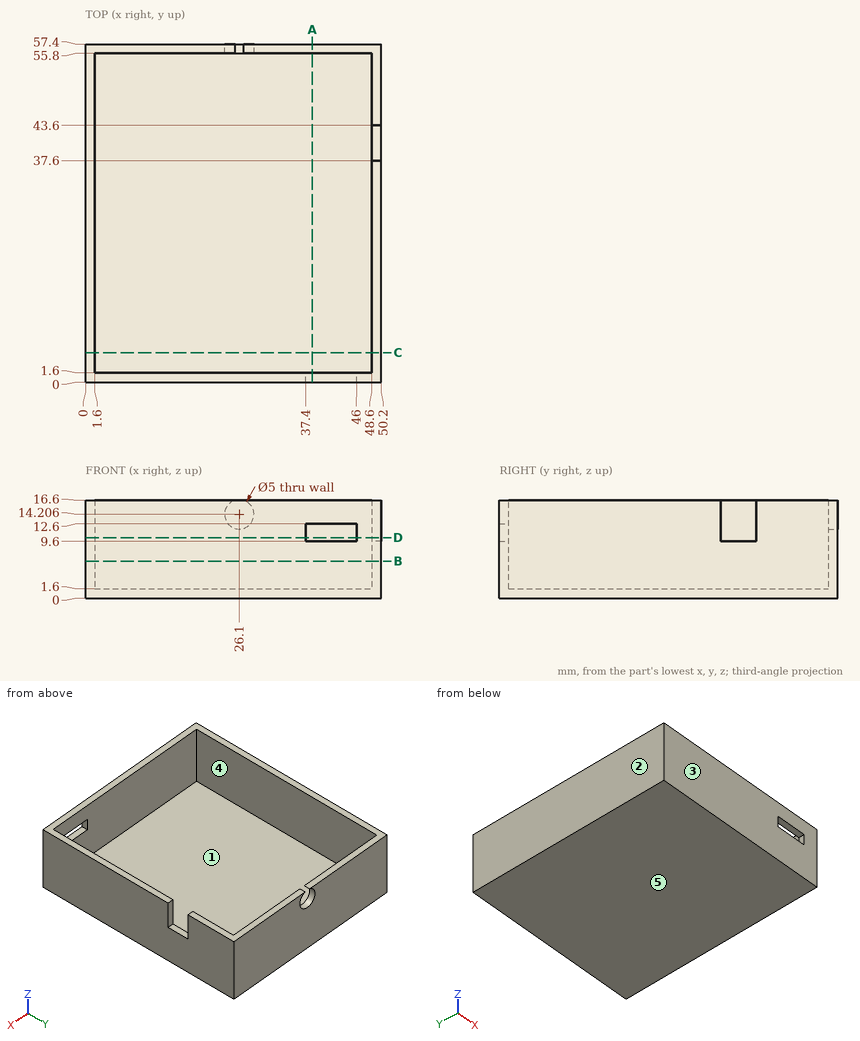
Study the drawing (mm; zero at the part's minimum x, y, z) and answer. A direction names the side the tool comes from. Give positions to 0.01 mm unless a question says otherwise; leave off trailing zeros. Write each loop counter-clockwise with the first axis right and the second up, starting at its lowest first coordinate (ties: lowest second). Pieces come first, ordered by that corner, then holes. Notation, with made-up numbers: (79, -30.5) -> (120, -30.5) arc R12 cw to (120, -24.5) -> close; hole circle Ø6 at (7, 11.5). An arc over 180 degrees is marked (long way). Answer as a JSON object with one key per item and string values. Group by question number.
1) Find section C-C (y = 5). Write down the section's boundary in (x, z), and give its area (3 significant figures).
2) Find section D-D (z = 10.25). Write down the section's boundary in (x, y).
3) Each of these flat-tipped pins is pushed along its axis until it touches: P1, Ø1.3, axis at x = 49, y = 41, coming from the +Z side; P2, Ø12, axis at x = 29.5, y = 9, coming from the +Z side. Where does it stop, or does it pass through?
4) Find section B-B (z = 6.25). Write down the section's boundary in (x, y), and give its area (3 significant figures).
5) Find section A-A (x = 38.5). Write down the section's boundary in (y, z).
6) Consider L1, parallel to Y at x = 23.5, z = 3.75; L2, parallel to X at y = 53, z = 2.75; L3, parallel to Z at x = 45, y = 20. Determine where each line is inside the solid, lowest interval first. Write a range as from..to.
7) A tool of negligible diameter and unlimited length cuts with its end or side. For the marked faces 4 and 5, from which of +Z, -Z, +X, -X, +Y, -Y can it reach the whole face along a straight path? Write none if from no direction.
8) The mould has two halves that part along Y. Classify the marked faces 1, 2 and 3: +Y half, -Y half, draft (parallel to the pull), parting line (faces both ways), or undercut.
Values follow:
{
 "1": {"outline": "(0, 0) -> (50.2, 0) -> (50.2, 16.6) -> (48.6, 16.6) -> (48.6, 1.6) -> (1.6, 1.6) -> (1.6, 16.6) -> (0, 16.6) -> close", "area": "128 mm2"},
 "2": {"outline": "(0, 0) -> (37.4, 0) -> (37.4, 1.6) -> (1.6, 1.6) -> (1.6, 55.8) -> (48.6, 55.8) -> (48.6, 43.6) -> (50.2, 43.6) -> (50.2, 57.4) -> (0, 57.4) -> close; (46, 0) -> (50.2, 0) -> (50.2, 37.6) -> (48.6, 37.6) -> (48.6, 1.6) -> (46, 1.6) -> close"},
 "3": {"P1": "stops at z = 9.6", "P2": "stops at z = 1.6"},
 "4": {"outline": "(0, 0) -> (50.2, 0) -> (50.2, 57.4) -> (0, 57.4) -> close; hole (1.6, 1.6) -> (48.6, 1.6) -> (48.6, 55.8) -> (1.6, 55.8) -> close", "area": "334 mm2"},
 "5": {"outline": "(0, 0) -> (57.4, 0) -> (57.4, 16.6) -> (55.8, 16.6) -> (55.8, 1.6) -> (1.6, 1.6) -> (1.6, 9.6) -> (0, 9.6) -> close; (0, 12.6) -> (1.6, 12.6) -> (1.6, 16.6) -> (0, 16.6) -> close"},
 "6": {"L1": "y = 0..1.6, 55.8..57.4", "L2": "x = 0..1.6, 48.6..50.2", "L3": "z = 0..1.6"},
 "7": {"face 4": "+Z", "face 5": "-Z, +X, -X, +Y, -Y"},
 "8": {"face 1": "undercut", "face 2": "draft", "face 3": "-Y half"}
}
